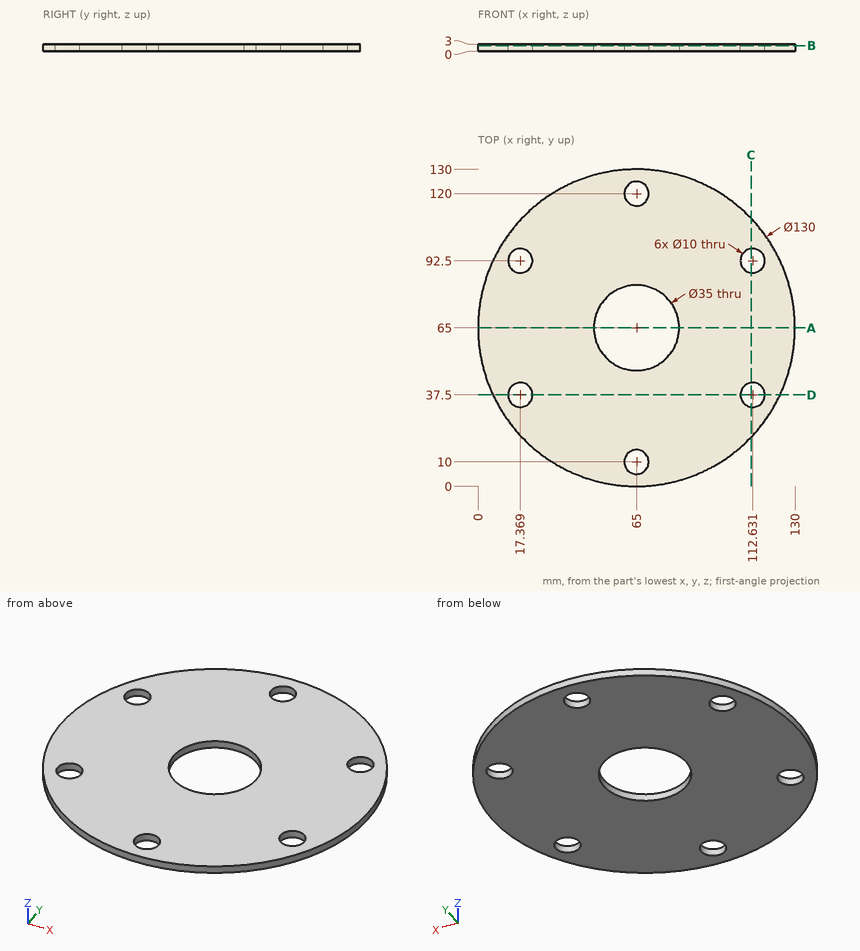
The figure shows three views and two pictorial views of one solid part (mm, origin at its lowest corner). Answer the questions. Coordinates: 2 decimals unless noted, no trailing zeros. Order: outer loops, then holes, each group sorted by start corner. A loop starts at its lowest first (then second) coordinate and runs counter-clockwise, first axis right, second up.
Q1. A cutting plane is placed at C-C, the plane x = 112. Write down the section's boundary in (y, z).
Q2. A cutting plane is placed at A-A, the plane y = 65. Write down the section's boundary in (x, z), and give its area (3 significant figures).
Q3. Given P1, Ø8, axis at x = 17.37, y = 92.5, coming from the -Z side; P2, Ø1.5, axis at x = 38.5, z = 2.5, coming from the +Y side; P3, Ø1.5, axis at x = 20, z = 2, coming from the +Y side, each flat-ended and moving along its own axis, determine where each tip first touches the part or whether it passes through.
Q4. A cutting plane is placed at B-B, the plane z = 2.35. Write down the section's boundary in (x, y), and give its area (3 significant figures).
Q5. Consider line 1 (Y direction, x = 65, z = 1.55); line 2 (X direction, y = 64, z = 1.5); line 3 (X direction, y = 90, z = 0.9). Determine where each line is inside the solid, lowest interval first.
Q6. A cutting plane is placed at D-D, the plane y = 37.5. Write down the section's boundary in (x, z).
Answers follow:
1. outline: (20.1, 0) - (32.54, 0) - (32.54, 3) - (20.1, 3) - close; (42.46, 0) - (87.54, 0) - (87.54, 3) - (42.46, 3) - close; (97.46, 0) - (109.9, 0) - (109.9, 3) - (97.46, 3) - close
2. outline: (0, 0) - (47.5, 0) - (47.5, 3) - (0, 3) - close; (82.5, 0) - (130, 0) - (130, 3) - (82.5, 3) - close
2. area: 285 mm2
3. P1: passes through
3. P2: stops at y = 124.68
3. P3: stops at y = 112.61
4. outline: circle Ø130 at (65, 65); hole circle Ø10 at (17.37, 37.5); hole circle Ø10 at (17.37, 92.5); hole circle Ø35 at (65, 65); hole circle Ø10 at (65, 10); hole circle Ø10 at (65, 120); hole circle Ø10 at (112.63, 37.5); hole circle Ø10 at (112.63, 92.5)
4. area: 11,800 mm2
5. line 1: y = 0 to 5, 15 to 47.5, 82.5 to 115, 125 to 130
5. line 2: x = 0.01 to 47.53, 82.47 to 129.99
5. line 3: x = 5 to 13.04, 21.7 to 108.3, 116.96 to 125
6. outline: (6.1, 0) - (12.37, 0) - (12.37, 3) - (6.1, 3) - close; (22.37, 0) - (107.63, 0) - (107.63, 3) - (22.37, 3) - close; (117.63, 0) - (123.9, 0) - (123.9, 3) - (117.63, 3) - close
